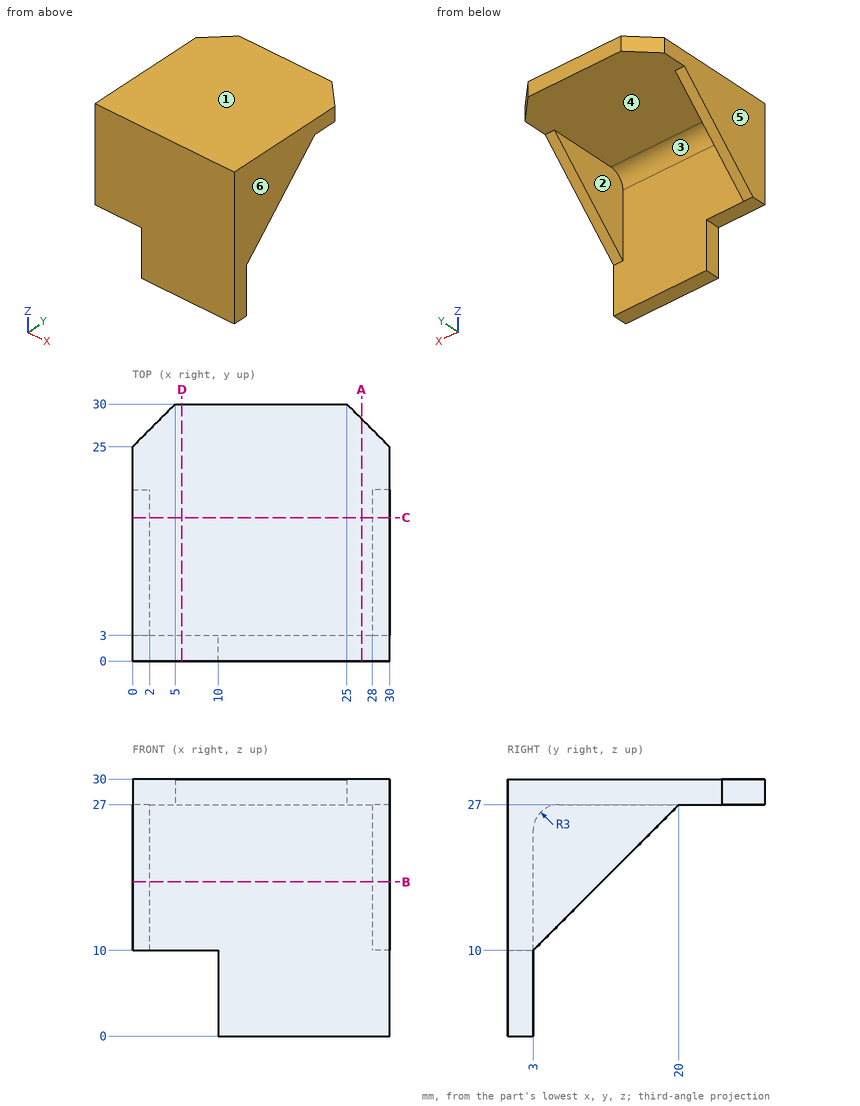
Answer from the drawing. Dimensions are ordinates in mm from the lowest x, y and z of the part. A direction names the side the tool comes from. Give positions to 0.01 mm unless a question says otherwise; leave off trailing zeros. Write each loop counter-clockwise with the first axis right and the second up, starting at its lowest first coordinate (ties: lowest second). Pieces come first, ordered by that corner, then holes. Notation, with made-up numbers: (-7, 37) - (6, 37) arc R23 ccw to (6, 50) - close; hole circle Ø5 at (-21.5, -18). An arc over 180 degrees is marked (long way). Answer in a Markdown table with one row per item. Add a question column.
Item 1: Section A-A, the plane x = 26.75 is taken. Write down the section's boundary in (y, z), and give its area (3 significant figures).
Item 2: A tool of negligible diameter and unlimited length cuts with its end or side. For the marked faces 1 and 2, from which of +Z, -Z, +X, -X, +Y, -Y can it reach the whole face along a straight path? Write none if from no direction.
Item 3: Find the intervals of material crossed by L1, parallel to X at y = 7.5, z = 19; L2, parallel to Z at x = 5.5, y = 1.5; L3, parallel to Y at x = 5.5, z = 16, in increasing order.
Item 4: Section C-C, the plane y = 16.75 is taken. Write down the section's boundary in (x, z).
Item 5: Determine the mould class of the marked faces 3, 4, 5 and 6 for opening direction X: pulls with the +X half, pulls with the -X half, needs draft (parallel to the pull), parting line crosses it, or undercut.
Item 6: Flat-ended cylindrical pins translate along their axes: P1, Ø7, axis at x = 11, y = 22.5, coming from the -Z side; P2, Ø1.5, axis at x = 5, y = 1, coming from the -Z side; P3, Ø12, axis at x = 11, z = 4.5, coming from the +Y side; P4, Ø5, axis at y = 19.5, z = 24, coming from the +X side. Find the tip coordinate at first contact, or state that the pin passes through.
Item 7: Section B-B, the plane z = 18 is taken. Write down the section's boundary in (x, y), and give its area (3 significant figures).
Item 8: Section D-D, the plane x = 5.75 is taken. Write down the section's boundary in (y, z), and give its area (3 significant figures).
Recorded:
| question | item | result |
|---|---|---|
| 1 | outline | (0, 0) - (3, 0) - (3, 24) arc R3 cw to (6, 27) - (28.25, 27) - (28.25, 30) - (0, 30) - close |
| 1 | area | 168 mm2 |
| 2 | face 1 | +Z, +X, -X, +Y, -Y |
| 2 | face 2 | -Z, +Y |
| 3 | L1 | x = 0 to 2, 28 to 30 |
| 3 | L2 | z = 10 to 30 |
| 3 | L3 | y = 0 to 3 |
| 4 | outline | (0, 23.75) - (2, 23.75) - (2, 27) - (28, 27) - (28, 23.75) - (30, 23.75) - (30, 30) - (0, 30) - close |
| 5 | face 3 | undercut |
| 5 | face 4 | undercut |
| 5 | face 5 | pulls with the -X half |
| 5 | face 6 | pulls with the +X half |
| 6 | P1 | stops at z = 27 |
| 6 | P2 | stops at z = 10 |
| 6 | P3 | stops at y = 3 |
| 6 | P4 | stops at x = 30 |
| 7 | outline | (0, 0) - (30, 0) - (30, 11) - (28, 11) - (28, 3) - (2, 3) - (2, 11) - (0, 11) - close |
| 7 | area | 122 mm2 |
| 8 | outline | (0, 10) - (3, 10) - (3, 24) arc R3 cw to (6, 27) - (30, 27) - (30, 30) - (0, 30) - close |
| 8 | area | 143 mm2 |
